from build123d import *

# Parameters (mm, degrees)
F0_W      = 180
F0_H      = 10
F1_DEPTH  = 15
F2_W      = 180
F2_H      = 10
F3_DEPTH  = 5
F4_W      = 5
F4_H      = 10
F5_DEPTH  = 5
F6_R      = 1.5
F7_DEPTH  = 25
F8_W      = 90
F8_H      = 10
F9_DEPTH  = 25
F10_W     = 5
F10_H     = 5
F11_DEPTH = 5


with BuildPart() as f1:
    # F0 (on Top) → F1 (new body)
    with BuildSketch(Plane.XY):
        Rectangle(F0_W, F0_H)
    extrude(amount=F1_DEPTH)

    # F2 (on face) → F3 (cut)
    with BuildSketch(Plane.XZ.offset(5)):
        with Locations((0, 10)):
            Rectangle(F2_W, F2_H)
    extrude(amount=-F3_DEPTH, mode=Mode.SUBTRACT)

    # F4 (on face) → F5 (join)
    with BuildSketch(Plane(origin=(-90, 0, 0), x_dir=(0, -1, 0), z_dir=(-1, 0, 0))):
        with Locations((-2.5, 10)):
            Rectangle(F4_W, F4_H)
    extrude(amount=F5_DEPTH)

    # F6 (on face) → F7 (cut)
    with BuildSketch(Plane.XZ):
        with Locations((-92.5, 7.5)):
            Circle(F6_R)
    extrude(amount=-F7_DEPTH, mode=Mode.SUBTRACT)

    # F8 (on face) → F9 (cut)
    with BuildSketch(Plane(origin=(0, 0, 0), x_dir=(1, 0, 0), z_dir=(0, 0, -1))):
        with Locations((45, 0)):
            Rectangle(F8_W, F8_H)
    extrude(amount=-F9_DEPTH, mode=Mode.SUBTRACT)

    # F10 (on face) → F11 (join)
    with BuildSketch(Plane(origin=(-95, 0, 0), x_dir=(0, -1, 0), z_dir=(-1, 0, 0))):
        Polygon((-5, 10), (-5, 15), (-10, 10), align=None)
        with Locations((2.5, 12.5)):
            Rectangle(F10_W, F10_H)
    extrude(amount=-F11_DEPTH)

    # F12: F1 across face


with BuildPart() as f1_1:
    add(f1.part)
    add(f1.part.mirror(Plane(origin=(0, 1.25, 6.25), x_dir=(0, 1, 0), z_dir=(1, 0, 0))))


solid = f1_1.part
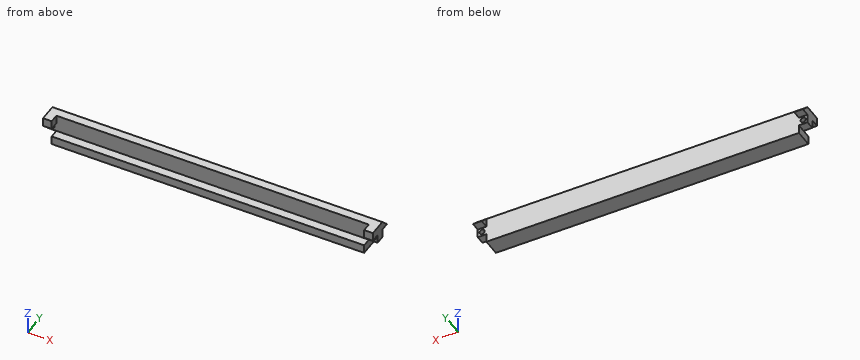
Verification items for the finished model (mm, model axes). Coordinates: 2 decimals unless noted, no trailing zeros. Order: outer loops, then holes, each group sorted by start corner. A loop starts at its lowest first (then second) coordinate and runs counter-clockwise, first axis right, second up. Notation, with made-up numbers: M 29.25,63.5 L 78.25,63.5 A19 ccw 78.25,77.5 Z; hole C -7,86 d1. An arc over 180 degrees is marked long. One line per item, written item: value. Start each with the question number.
Item 1: Depth check by flat-ended pin: P1, Ø1.5, axis at y = -3, z = 8, coming from the +X side; P2, Ø1.5, axis at x = -91.5, y = -2.5, coming from the -Z side; P3, Ø5, axis at x = 49.5, z = 9.5, coming from the +Y side; P4, Ø1.5, axis at x = -33.5, y = -2.5, coming from the +Z side. Enter the tip coordinate at first touch or a pass-through.
Item 2: Sectioned sample at A-A on x = 23. Record the cut outline in (y, z).
Item 3: Sectioned sample at B-B on z = 2.5. Record the cut outline in (x, y), then the cut area to 3 significant figures.
Item 4: Thickness scan on probe 1 along Z at (x, y) = (-92.5, 1.7); probe 2 along X at (y, z) = (-1.5, 13.25); probe 3 along Y at (x, z) = (-87, 10.5). Record the ranges inside material, lowest first.
Calculated:
1. P1: through
1. P2: z = 10
1. P3: y = 5
1. P4: z = 5
2. outline: M -5,0 L 5,0 L 5,15 L 0,15 L 0,5 L -5,5 Z
3. outline: M -90,-5 L 90,-5 L 90,5 L -90,5 Z
3. area: 1,800 mm^2
4. probe 1: 5 to 6, 9 to 15
4. probe 2: -95 to -90, 90 to 95
4. probe 3: 0 to 5
